from build123d import *

# Parameters (mm, degrees)
SKIZZE1_W                                            = 140
SKIZZE1_H                                            = 10
AUFSATZ_LINEAR_AUSTRAGEN1_DEPTH                      = 15
SCHNITT_LINEAR_AUSTRAGEN1_DEPTH                      = 15
FORMSENKUNG_F_R_M4_SENKSCHRAUBE_MIT_INNE_D           = 4.5
FORMSENKUNG_F_R_M4_SENKSCHRAUBE_MIT_INNE_CSINK_D     = 9.18
FORMSENKUNG_F_R_M4_SENKSCHRAUBE_MIT_INNE_CSINK_ANGLE = 90


with BuildPart() as part:
    # Skizze1 → Aufsatz-Linear austragen1 (new body)
    with BuildSketch(Plane(origin=(0, 0, 0), x_dir=(1, 0, 0), z_dir=(0, 1, 0))):
        with Locations((93.874498843, 0.286555153)):
            Rectangle(SKIZZE1_W, SKIZZE1_H)
    extrude(amount=AUFSATZ_LINEAR_AUSTRAGEN1_DEPTH)

    # Skizze2 → Schnitt-Linear austragen1 (cut)
    with BuildSketch(Plane(origin=(0, 0, -5.286555153), x_dir=(-1, 0, 0), z_dir=(0, 0, -1))):
        with BuildLine():
            Line((-37.124498843, 8), (-37.124498843, 0))
            Line((-37.124498843, 0), (-30.624498843, 0))
            Line((-30.624498843, 0), (-30.624498843, 8))
            ThreePointArc((-30.624498843, 8), (-33.874498843, 11.25), (-37.124498843, 8))
        make_face()
        with BuildLine():
            Line((-157.124498843, 8), (-157.124498843, -0.120378635))
            Line((-157.124498843, -0.120378635), (-150.624498843, -0.120378635))
            Line((-150.624498843, -0.120378635), (-150.624498843, 8))
            ThreePointArc((-150.624498843, 8), (-153.874498843, 11.25), (-157.124498843, 8))
        make_face()
    extrude(amount=-SCHNITT_LINEAR_AUSTRAGEN1_DEPTH, mode=Mode.SUBTRACT)

    # Formsenkung für M4 Senkschraube mit Innensechskant1 (through all)
    with Locations(Plane(origin=(82.249498843, 0, 0), x_dir=(0, 0, -1), z_dir=(0, -1, 0))):
        with Locations((0, 0), (0, 23.25)):
            CounterSinkHole(FORMSENKUNG_F_R_M4_SENKSCHRAUBE_MIT_INNE_D / 2, FORMSENKUNG_F_R_M4_SENKSCHRAUBE_MIT_INNE_CSINK_D / 2, counter_sink_angle=FORMSENKUNG_F_R_M4_SENKSCHRAUBE_MIT_INNE_CSINK_ANGLE)


solid = part.part
Work out the finished part from the listing and answer in its coordinate system (mm). A direction names the side the tool comes from. Give positions to 0.01 mm unless a question says otherwise; leave off trailing zeros. Loops run counter-clockwise (first coordinate to the right, second up) from the corner with the lowest first, then second, coordinate; pieces in that order, holes last. Notation, with made-up numbers: M 26.5,82 L 44.5,82 A17 cw 44.5,114 Z; hole C -9.5,63.5 d1. An arc over 180 degrees is marked long. Use CSV: the item, a comma, the result in double quotes.
1) Find section A-A on z = 0. Write down the section's boundary in (x, y).
Answer:
outline,"M 23.87,0 L 30.62,0 L 30.62,8 A3.25 cw 37.12,8 L 37.12,0 L 77.66,0 L 80,2.34 L 80,15 L 23.87,15 Z; M 84.5,2.34 L 86.84,0 L 100.91,0 L 103.25,2.34 L 103.25,15 L 84.5,15 Z; M 107.75,2.34 L 110.09,0 L 150.62,0 L 150.62,8 A3.25 cw 157.12,8 L 157.12,0 L 163.87,0 L 163.87,15 L 107.75,15 Z"
2) Find section B-B on y = 4.5. Write down the section's boundary in (x, z).
Answer:
outline,"M 23.87,-5.29 L 30.62,-5.29 L 30.62,4.71 L 23.87,4.71 Z; M 37.12,-5.29 L 150.62,-5.29 L 150.62,4.71 L 37.12,4.71 Z; M 157.12,-5.29 L 163.87,-5.29 L 163.87,4.71 L 157.12,4.71 Z; hole C 82.25,0 d4.5; hole C 105.5,0 d4.5"
3) Which of the six approach directions +Z, -Z, +X, -X, +Y, -Y give full straight-line access (tool end or side, diameter ignored) to faces 4 (the flat face through (93, 15, 0)), 5 (the flat face through (30.624, 4, 0))?
Answer:
face 4,"+Z, -Z, +X, -X, +Y"
face 5,"+Z, -Z, -Y"
4) Consider L1, parallel to X at y = 11.5, z = 0; L2, parallel to X at y = 6, z = 4; L3, parallel to X at y = 7.5, z = 0. Determine where each line is inside the solid, lowest interval first.
Answer:
L1,"23.87 to 80, 84.5 to 103.25, 107.75 to 163.87"
L2,"23.87 to 30.62, 37.12 to 150.62, 157.12 to 163.87"
L3,"23.87 to 30.62, 37.12 to 80, 84.5 to 103.25, 107.75 to 150.62, 157.12 to 163.87"
5) Determine the mould class of faces 1 (the cylindrical face through (107.73, 8.76, -0.29)), 2 (the flat face through (93, 7, -5.287)), 3 (the flat face through (157.124, 4, 0)) for opening direction Z: released by +Z, released by -Z, zero draft, split by the parting line, or undercut.
Answer:
face 1,"undercut"
face 2,"released by -Z"
face 3,"zero draft"
6) Find section C-C on y = 13.5. Write down the section's boundary in (x, z).
Answer:
outline,"M 23.87,-5.29 L 163.87,-5.29 L 163.87,4.71 L 23.87,4.71 Z; hole C 82.25,0 d4.5; hole C 105.5,0 d4.5"
